Input: part model. Units: mm. Frame: model coordinates. Face numbers are marked on the shaded views. A direction names the side the tool comes from. Coordinates: 2 decimals unless noted, no trailing zeros. Write each loop counter-clockwise with the first axis right and the second up, starting at its lowest first coordinate (ties: lowest second). Pieces come first, ordered by that corner, then holes. Notation, with made-up numbers: (66.25, -30) - (79.25, -30) arc R14 cw to (79.25, -4) - close; hole circle Ø6 at (85.5, -31). An arc over 180 degrees is marked (long way). Use a Markdown table: item, result. Add a question column.
Q1. Mould query, pull axis Y, two halves, no side actions, for the marked faces 1, 2, 3 and 4. Classes: released by +Y, released by -Y, zero draft, split by the parting line, or undercut.
Q2. Section query A-A (z = -12). Return the cut outline in (x, y), then the cut area to 3 significant figures.
Q3. Section query B-B (x = -85.25). Return the cut outline in (y, z).
Q4. Material intervals for probe 1 along Z at (x, y) = (-83.75, -24); probe 2 along Y at (x, z) = (-87, -1.25); probe 3 along X at (y, z) = (-4, -16.5), sorted ascending. Write a range as from..to.
Q5. Section query D-D (x = -88.5). Return the cut outline in (y, z).
Q6. Pin query (flat end, axial travel): P1, Ø8, axis at x = -90.5, z = -11, coming from the -Y side; P2, Ø10, axis at y = 10.5, z = -16.5, coming from the +X side; P3, Ø3, axis at x = -87, z = -18, coming from the +Y side. Return the tip coordinate at first contact, or that it passes through.
Q7. Section query C-C (z = -3.75). Return the cut outline in (x, y).
Q8. Set-up query: the marked faces 5, 6, 7 and 8. Return all of +Z, -Z, +X, -X, +Y, -Y with unobstructed straight access to the full face (end or side cutting, diameter ignored); none if empty.
from build123d import *

# Parameters (mm, degrees)
BOSS_EXTRUDE1_DEPTH = 20
SKETCH2_R           = 2.15
CUT_EXTRUDE1_DEPTH  = 5


with BuildPart() as part:
    # Sketch1 → Boss-Extrude1 (new body)
    with BuildSketch(Plane.XY):
        Polygon((-80.653583913, 18.961055491), (-76.668805121, 18.61243252), (-77.793114202, 5.761520915), (-87.256963834, 6.589500471), (-89.017509838, -13.533632431), (-79.553660206, -14.361611987), (-80.677969287, -27.212523592), (-84.662748079, -26.863900621), (-83.878346395, -17.898148338), (-93.342196027, -17.070168782), (-90.90183523, 10.823282764), (-81.437985598, 9.995303208), align=None)
    extrude(amount=-BOSS_EXTRUDE1_DEPTH)

    # Sketch2 → Cut-Extrude1 (cut)
    with BuildSketch(Plane(origin=(-81.687205696, 7.146704453, 0), x_dir=(0, 0, 1), z_dir=(-0.996194698, 0.087155743, 0))):
        with Locations((-4, -30.140520061)):
            Circle(SKETCH2_R)
        with Locations((-16, -30.140520061)):
            Circle(SKETCH2_R)
        with Locations((-4, 7.859479939)):
            Circle(SKETCH2_R)
        with Locations((-16, 7.859479939)):
            Circle(SKETCH2_R)
    extrude(amount=-CUT_EXTRUDE1_DEPTH, mode=Mode.SUBTRACT)


solid = part.part
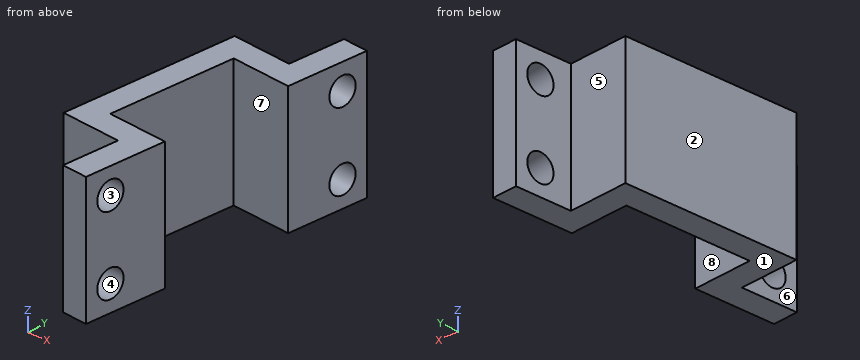
Values follow:
| question | item | result |
|---|---|---|
| 1 | face 1 | zero draft |
| 1 | face 2 | released by +Y |
| 1 | face 3 | undercut |
| 1 | face 4 | undercut |
| 2 | outline | (-93.34, -17.07) - (-83.88, -17.9) - (-84.66, -26.86) - (-80.68, -27.21) - (-79.55, -14.36) - (-89.02, -13.53) - (-87.26, 6.59) - (-77.79, 5.76) - (-76.67, 18.61) - (-80.65, 18.96) - (-81.44, 10) - (-90.9, 10.82) - close |
| 2 | area | 258 mm2 |
| 3 | outline | (-17.78, -20) - (-13.86, -20) - (-13.86, 0) - (-17.78, 0) - close; (6.41, -20) - (10.33, -20) - (10.33, 0) - (6.41, 0) - close |
| 4 | probe 1 | -20..-17.87, -14.13..-5.87, -2.13..0 |
| 4 | probe 2 | -17.63..-13.71, 6.57..10.48 |
| 4 | probe 3 | -92.2..-88.18 |
| 5 | outline | (-17.49, -20) - (-13.58, -20) - (-13.58, 0) - (-17.49, 0) - close; (-7.62, -20) - (10.61, -20) - (10.61, 0) - (-7.62, 0) - close |
| 6 | P1 | y = -17.67 |
| 6 | P2 | x = -76.96 |
| 6 | P3 | y = 10.61 |
| 7 | outline | (-93.34, -17.07) - (-83.88, -17.9) - (-84.13, -20.75) - (-80.14, -21.1) - (-79.55, -14.36) - (-89.02, -13.53) - (-87.26, 6.59) - (-77.79, 5.76) - (-77.2, 12.5) - (-81.19, 12.85) - (-81.44, 10) - (-90.9, 10.82) - close; (-84.66, -26.86) - (-80.68, -27.21) - (-80.52, -25.36) - (-84.5, -25.01) - close; (-80.82, 17.1) - (-76.83, 16.75) - (-76.67, 18.61) - (-80.65, 18.96) - close |
| 8 | face 5 | +Z, -Z, +Y |
| 8 | face 6 | +Z, -Z, -X |
| 8 | face 7 | +Z, -Z |
| 8 | face 8 | +Z, -Z, +X |
